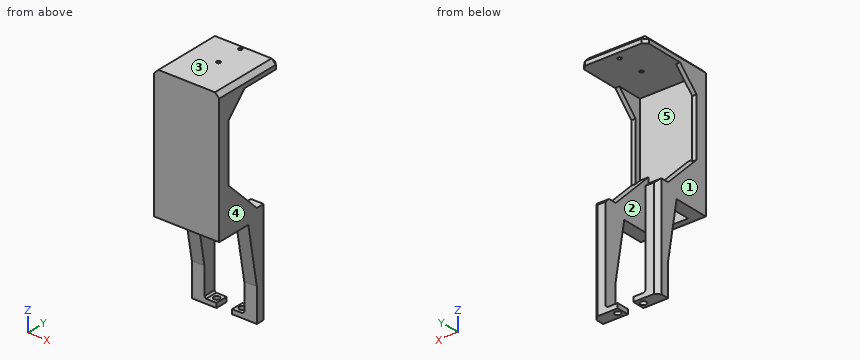
from build123d import *

# Parameters (mm, degrees)
SKETCH1_R             = 1.45
BOSS_EXTRUDE1_DEPTH   = 2.2
BOSS_EXTRUDE1_2_DEPTH = 2.2
SKETCH8_W             = 6
SKETCH8_H             = 5.9
BOSS_EXTRUDE6_DEPTH   = 42
BOSS_EXTRUDE7_DEPTH   = 5
SKETCH10_W            = 31
SKETCH10_H            = 3
BOSS_EXTRUDE8_DEPTH   = 53.85
SKETCH11_W            = 31
SKETCH11_H            = 35.214875224
SKETCH11_R            = 0.925
BOSS_EXTRUDE9_DEPTH   = 4
CHAMFER6_SIZE         = 19.1
CHAMFER7_SIZE         = 12
CHAMFER8_SIZE         = 2
CUT_EXTRUDE2_START    = 2
CUT_EXTRUDE2_DEPTH    = 27
CHAMFER10_SIZE        = 0.8
SKETCH14_W            = 7.5
SKETCH14_H            = 5.9
CUT_EXTRUDE3_DEPTH    = 112.547893301
CHAMFER11_SIZE        = 5
CHAMFER11_SIZE2       = 28.356409098
SKETCH15_W            = 2
SKETCH15_H            = 27.75
BOSS_EXTRUDE10_DEPTH  = 2.5


with BuildPart() as part:
    # Sketch1 → Boss-Extrude1 (new body)
    with BuildSketch(Plane.XY):
        Polygon((0, 0), (0, 5.9), (12.25, 5.9), (12.25, 0), (2.5, 0), align=None)
        with Locations((9.4, 2.95)):
            Circle(SKETCH1_R, mode=Mode.SUBTRACT)
    extrude(amount=BOSS_EXTRUDE1_DEPTH)



with BuildPart() as body_2:
    # Sketch1 → Boss-Extrude1 2 (new body)
    with BuildSketch(Plane.XY):
        Polygon((31, 0), (31, 5.9), (18.75, 5.9), (18.75, 0), (28.5, 0), align=None)
        with Locations((21.6, 2.95)):
            Circle(SKETCH1_R, mode=Mode.SUBTRACT)
    extrude(amount=BOSS_EXTRUDE1_2_DEPTH)


with BuildPart() as part_1:
    add(part.part)

    add(body_2.part)  # Boss-Extrude6 merges body 2
    # Sketch8 → Boss-Extrude6 (add)
    with BuildSketch(Plane.XY.offset(2.2)):
        with Locations((3, 2.95)):
            Rectangle(SKETCH8_W, SKETCH8_H)
        with Locations((28, 2.95)):
            Rectangle(SKETCH8_W, SKETCH8_H)
    extrude(amount=BOSS_EXTRUDE6_DEPTH)

    # Sketch9 → Boss-Extrude7 (add)
    with BuildSketch(Plane.XY.offset(44.2)):
        Polygon((0, 5.9), (0, -22.1), (31, -22.1), (31, 5.9), (25, 5.9), (25, -19.1), (6, -19.1), (6, 5.9), align=None)
    extrude(amount=BOSS_EXTRUDE7_DEPTH)

    # Sketch10 → Boss-Extrude8 (add)
    with BuildSketch(Plane.XY.offset(49.2)):
        with Locations((15.5, -20.6)):
            Rectangle(SKETCH10_W, SKETCH10_H)
    extrude(amount=BOSS_EXTRUDE8_DEPTH)

    # Sketch11 → Boss-Extrude9 (add)
    with BuildSketch(Plane.XY.offset(103.05)):
        with Locations((15.5, -4.492562388)):
            Rectangle(SKETCH11_W, SKETCH11_H)
        with Locations((15.5, -3.45)):
            Circle(SKETCH11_R, mode=Mode.SUBTRACT)
        with Locations(Location((15.5, 9.35, 0), (0, 0, 180))):
            Circle(SKETCH11_R, mode=Mode.SUBTRACT)
    extrude(amount=BOSS_EXTRUDE9_DEPTH)

    # Chamfer6
    chamfer6_edges = [part_1.edges().sort_by_distance(p)[0] for p in [
        (3, -19.1, 49.2),
        (28, -19.1, 49.2),
    ]]
    chamfer(chamfer6_edges, length=CHAMFER6_SIZE)

    # Chamfer7
    chamfer7_edges = [part_1.edges().sort_by_distance(p)[0] for p in [
        (15.5, -19.1, 103.05),
    ]]
    chamfer(chamfer7_edges, length=CHAMFER7_SIZE)

    # Chamfer8
    chamfer8_edges = [part_1.edges().sort_by_distance(p)[0] for p in [
        (0, -4.492562388, 107.05),
        (31, -4.492562388, 107.05),
        (15.5, 13.114875224, 107.05),
        (0, 13.114875224, 105.05),
        (31, 13.114875224, 105.05),
        (31, 5.9, 24.6),
        (3, 5.9, 49.2),
        (28, 5.9, 49.2),
        (0, 5.9, 24.6),
    ]]
    chamfer(chamfer8_edges, length=CHAMFER8_SIZE)

    # Sketch13 → Cut-Extrude2 (cut)
    with BuildSketch(Plane(origin=(0, 0, 0), x_dir=(0, 0, -1), z_dir=(1, 0, 0)).offset(CUT_EXTRUDE2_START)):
        Polygon((-103.05, -7.1), (-91.05, -19.1), (-103.05, -19.1), align=None)
    extrude(amount=CUT_EXTRUDE2_DEPTH, mode=Mode.SUBTRACT)

    # Chamfer10
    chamfer10_edges = [part_1.edges().sort_by_distance(p)[0] for p in [
        (6, 2.95, 2.2),
        (25, 2.95, 2.2),
    ]]
    chamfer(chamfer10_edges, length=CHAMFER10_SIZE)

    # Sketch14 → Cut-Extrude3 (cut, through all)
    with BuildSketch(Plane.XY.offset(2.2)):
        with Locations((15.5, 2.95)):
            Rectangle(SKETCH14_W, SKETCH14_H)
    extrude(amount=-CUT_EXTRUDE3_DEPTH, mode=Mode.SUBTRACT)

    # Chamfer11
    chamfer11_edges = [part_1.edges().sort_by_distance(p)[0] for p in [
        (3, 0, 44.2),
        (28, 0, 44.2),
    ]]
    chamfer11_side = [part_1.faces().sort_by_distance(p)[0] for p in [
        (3, -0.380711177, 44.2),
    ]]
    chamfer(chamfer11_edges, length=CHAMFER11_SIZE, length2=CHAMFER11_SIZE2, reference=chamfer11_side[0])

    # Sketch15 → Boss-Extrude10 (add)
    with BuildSketch(Plane(origin=(0, -19.1, 0), x_dir=(1, 0, 0), z_dir=(0, 1, 0))):
        with Locations((1, -79.675)):
            Rectangle(SKETCH15_W, SKETCH15_H)
        with Locations((30, -79.675)):
            Rectangle(SKETCH15_W, SKETCH15_H)
    extrude(amount=BOSS_EXTRUDE10_DEPTH)


solid = part_1.part
Build history of the part. All positions in model axes, mm. Face numbers are marked on the shaded views. A direction names the side the tool comes from. Round coordinates to 2 decimals unless told otherwise and drop trailing zeros. Write each loop counter-clockwise with the first axis right and the second up, starting at its lowest first coordinate (ties: lowest second). Pieces come first, ordered by that corner, then holes. Notation, with made-up numbers: (-20, -40) - (7, -40) arc R34 ccw to (7, -5) - close; hole circle Ø3 at (-10.75, -31). An arc over 180 degrees is marked (long way). One line per question, with ' | ' between items.
1. Mould opens along X. For the marked faces 1, 2 and 3 say: released by +X, released by -X, zero draft, split by the parting line, or undercut.
Results are:
face 1: released by -X | face 2: undercut | face 3: zero draft
2. Tool access for the marked faces 4 and 5: list every direction of +Z, -Z, +X, -X, +Y, -Y with a clear straight run to the whole face (end or side of a thin tool).
Results are:
face 4: +Z, -Z, +X, +Y, -Y | face 5: +Y
3. Band-saw the part on A-A, the plane y = 2.95. Write the cut outline in (x, z).
Results are:
outline: (0, 0) - (7.95, 0) - (7.95, 2.2) - (6.8, 2.2) - (6, 3) - (6, 49.2) - (0, 49.2) - close; (0, 103.05) - (31, 103.05) - (31, 105.05) - (29, 107.05) - (2, 107.05) - (0, 105.05) - close; (10.85, 0) - (11.75, 0) - (11.75, 2.2) - (10.85, 2.2) - close; (19.25, 0) - (20.15, 0) - (20.15, 2.2) - (19.25, 2.2) - close; (23.05, 0) - (31, 0) - (31, 49.2) - (25, 49.2) - (25, 3) - (24.2, 2.2) - (23.05, 2.2) - close
4. Band-saw the part on D-D, the plane z = 100.5. Write the cut outline in (x, y), and give its area (3 significant figures).
Results are:
outline: (0, -22.1) - (31, -22.1) - (31, -9.65) - (29, -9.65) - (29, -19.1) - (2, -19.1) - (2, -9.65) - (0, -9.65) - close | area: 131 mm^2
5. Drill centre lines: line 1 along X through (y, z) = (2, 1); line 2 along Y through (x, z) = (9.4, 0.65); line 3 along Z through (x, y) = (11.5, 5). Where is each one in solid material? Low to high. Write a range as from..to.
Results are:
line 1: 0..8.3, 10.5..11.75, 19.25..20.5, 22.7..31 | line 2: 0..1.5, 4.4..5.9 | line 3: 0..2.2, 103.05..107.05
6. Band-saw the part on C-C, the plane x = 21.6. Write the cut outline in (y, z), and give its area (3 significant figures).
Results are:
outline: (-22.1, 44.2) - (-19.1, 44.2) - (-19.1, 103.05) - (13.11, 103.05) - (13.11, 105.05) - (11.11, 107.05) - (-22.1, 107.05) - close; (0, 0) - (1.5, 0) - (1.5, 2.2) - (0, 2.2) - close; (4.4, 0) - (5.9, 0) - (5.9, 2.2) - (4.4, 2.2) - close | area: 322 mm^2
7. Band-saw the part on B-B, the plane y = -9.5. Write the cut outline in (x, z), and give its area (3 significant figures).
Results are:
outline: (0, 44.2) - (6, 44.2) - (6, 58.7) - (0, 58.7) - close; (0, 100.65) - (2, 100.65) - (2, 103.05) - (29, 103.05) - (29, 100.65) - (31, 100.65) - (31, 105.05) - (29, 107.05) - (2, 107.05) - (0, 105.05) - close; (25, 44.2) - (31, 44.2) - (31, 58.7) - (25, 58.7) - close | area: 304 mm^2
8. Drop flat-ended pins along their axis: pin 1 Ø3 at (x, z) = (9.5, 54.5) entering from +Y; pin 2 Ø1 at (x, z) = (29.5, 78.5) entering from +Y; pin 3 Ø13 at (x, z) = (7.5, 7) entering from -Y. Give the stop position or say it passes through.
Results are:
pin 1: y = -19.1 | pin 2: y = -16.6 | pin 3: y = 0
